For this review, take the finished solid that the model builds, in its own axes (mm). A direction names the side the tool comes from. Give positions to 0.01 mm unless a question says otherwise; leave off trailing zeros.
```python
from build123d import *

# Parameters (mm, degrees)
SKETCH1_W           = 75
SKETCH1_H           = 235.4
BOSS_EXTRUDE1_DEPTH = 5.7
SKETCH2_W           = 10
SKETCH2_H           = 5.7
CUT_EXTRUDE1_DEPTH  = 5.7
CUT_EXTRUDE2_DEPTH  = 5.7
SKETCH4_W           = 3
SKETCH4_H           = 224
CUT_EXTRUDE3_DEPTH  = 0.7


with BuildPart() as part:
    # Sketch1 → Boss-Extrude1 (new body)
    with BuildSketch(Plane.XY):
        with Locations((37.5, 117.7)):
            Rectangle(SKETCH1_W, SKETCH1_H)
    extrude(amount=BOSS_EXTRUDE1_DEPTH)

    # Sketch2 → Cut-Extrude1 (cut)
    with BuildSketch(Plane(origin=(0, 0, 0), x_dir=(-1, 0, 0), z_dir=(0, 0, -1))):
        with Locations((-70, 2.85)):
            Rectangle(SKETCH2_W, SKETCH2_H)
        with Locations((-5, 2.85)):
            Rectangle(SKETCH2_W, SKETCH2_H)
        with Locations((-5, 232.55)):
            Rectangle(SKETCH2_W, SKETCH2_H)
        with Locations((-70, 232.55)):
            Rectangle(SKETCH2_W, SKETCH2_H)
    extrude(amount=-CUT_EXTRUDE1_DEPTH, mode=Mode.SUBTRACT)

    # Sketch3 → Cut-Extrude2 (cut)
    with BuildSketch(Plane.XY.offset(5.7)):
        Polygon((65, 195), (63.55777949, 195), (25, 137.163330765), (25, 135), (26.44222051, 135), (65, 192.836669235), align=None)
        Polygon((60.67777949, 195), (57.79777949, 195), (25, 145.803330765), (25, 141.483330765), align=None)
        Polygon((54.91777949, 195), (52.03777949, 195), (25, 154.443330765), (25, 150.123330765), align=None)
        Polygon((49.15777949, 195), (46.27777949, 195), (25, 163.083330765), (25, 158.763330765), align=None)
        Polygon((43.39777949, 195), (40.51777949, 195), (25, 171.723330765), (25, 167.403330765), align=None)
        Polygon((37.63777949, 195), (34.75777949, 195), (25, 180.363330765), (25, 176.043330765), align=None)
        Polygon((31.87777949, 195), (28.99777949, 195), (25, 189.003330765), (25, 184.683330765), align=None)
        Polygon((65, 184.196669235), (65, 188.516669235), (29.32222051, 135), (32.20222051, 135), align=None)
        Polygon((65, 175.556669235), (65, 179.876669235), (35.08222051, 135), (37.96222051, 135), align=None)
        Polygon((65, 166.916669235), (65, 171.236669235), (40.84222051, 135), (43.72222051, 135), align=None)
        Polygon((65, 158.276669235), (65, 162.596669235), (46.60222051, 135), (49.48222051, 135), align=None)
        Polygon((65, 149.636669235), (65, 153.956669235), (52.36222051, 135), (55.24222051, 135), align=None)
        Polygon((65, 140.996669235), (65, 145.316669235), (58.12222051, 135), (61.00222051, 135), align=None)
    extrude(amount=-CUT_EXTRUDE2_DEPTH, mode=Mode.SUBTRACT)

    # Sketch4 → Cut-Extrude3 (cut)
    with BuildSketch(Plane.XY.offset(5.7)):
        with Locations((3.5, 117.7)):
            Rectangle(SKETCH4_W, SKETCH4_H)
    extrude(amount=-CUT_EXTRUDE3_DEPTH, mode=Mode.SUBTRACT)


solid = part.part
```
Item 1: Take a section at A-A on z = 1.1. State how many separate pieces and enclosed holes the cut face has, and give its area (3 significant figures).
Answer:
separate pieces: 1
enclosed holes: 13
area: 16,200 mm2
Item 2: Tool access review of faces 1 (the flat face through (57.132, 146.475, 2.89)), 2 (the flat face through (0, 116, 3)), 3 (the flat face through (70, 5.7, 3)): name each direction out of +Z, -Z, +X, -X, +Y, -Y from which nothing blocks a thin tool from reaching the whole face with its end or side.
Answer:
face 1: +Z, -Z
face 2: +Z, -Z, -X, +Y, -Y
face 3: +Z, -Z, +X, -Y
Item 3: The part is to be moulded in two halves that separate along X. For faces 4 (the flat face through (65, 143, 3)), 5 (the flat face through (40, 119, 5.7)), 6 (the flat face through (65, 233, 3)), say which applies: released by +X, released by -X, zero draft, split by the parting line, or undercut.
Answer:
face 4: undercut
face 5: zero draft
face 6: released by +X
Item 4: For L1, parallel to X at y = 26, z = 5.25; L2, parallel to Y at x = 70.5, z = 4.35, list the stretches that pass through material, from the lowest coordinate up.
Answer:
L1: x = 0 to 2, 5 to 75
L2: y = 5.7 to 229.7
